```python
from build123d import *

# Parameters (mm, degrees)
F0_W     = 40
F0_H     = 20
F1_DEPTH = 10
F2_W     = 9.5
F2_H     = 8.5
F3_DEPTH = 10
F4_R     = 2
F5_DEPTH = 10
F6_W     = 40
F6_H     = 2
F7_DEPTH = 3


with BuildPart() as f1:
    # F0 (on Top) → F1 (new body)
    with BuildSketch(Plane.XY):
        Rectangle(F0_W, F0_H)
    extrude(amount=F1_DEPTH)

    # F2 (on face) → F3 (join)
    with BuildSketch(Plane.XY.offset(10)):
        with Locations((0, -5.75)):
            Rectangle(F2_W, F2_H)
    extrude(amount=F3_DEPTH)

    # F4 (on face) → F5 (cut)
    with BuildSketch(Plane.XZ.offset(10)):
        with Locations((0, 15)):
            Circle(F4_R)
    extrude(amount=-F5_DEPTH, mode=Mode.SUBTRACT)

    # F6 (on face) → F7 (cut)
    with BuildSketch(Plane(origin=(0, 10, 0), x_dir=(-1, 0, 0), z_dir=(0, 1, 0))):
        with Locations((0, 4.25)):
            Rectangle(F6_W, F6_H)
    extrude(amount=-F7_DEPTH, mode=Mode.SUBTRACT)


solid = f1.part
```
Work out the finished part from the listing and answer in its coordinate system (mm). A direction names the side the tool comes from. Round coordinates to 2 decimals unless told otherwise and drop trailing zeros. Write each loop counter-clockwise with the first axis right and the second up, starting at its lowest first coordinate (ties: lowest second). Pieces come first, ordered by that corner, then holes. Notation, with made-up numbers: (20, 42) -> (78, 42) arc R5 ccw to (78, 51) -> close; hole circle Ø9 at (-20, 51.5). An arc over 180 degrees is marked (long way). Write each question's results on one line, items separated by ' | '.
1) For a pull along Z with two mould halves and no side action, classify faces 1 (the flat face through (-4.75, -6, 15)), 2 (the flat face through (0, -6, 20)), 3 (the flat face through (0, 9, 5.25)), 4 (the flat face through (0, 0, 0)) as +Z half, -Z half, draft (parallel to the pull), parting line (faces both ways), or undercut.
Findings:
face 1: draft | face 2: +Z half | face 3: undercut | face 4: -Z half
2) Which of the six approach directions +Z, -Z, +X, -X, +Y, -Y give full straight-line access (tool end or side, diameter ignored) to faces 5 (the flat face through (0, 9, 3.25)), 6 (the flat face through (-2.2, -1.5, 14.9)), 7 (the flat face through (4.75, -6, 15))?
Findings:
face 5: +X, -X, +Y | face 6: +Z, +X, -X, +Y | face 7: +Z, +X, +Y, -Y
3) The part is cut by section A-A (x = 0). Write down the section's boundary in (y, z), and give its area (3 significant figures).
Findings:
outline: (-10, 0) -> (10, 0) -> (10, 3.25) -> (7, 3.25) -> (7, 5.25) -> (10, 5.25) -> (10, 10) -> (-1.5, 10) -> (-1.5, 13) -> (-10, 13) -> close; (-10, 17) -> (-1.5, 17) -> (-1.5, 20) -> (-10, 20) -> close | area: 245 mm²
4) Flat-ended cylindrical pins translate along their axes: pin 1 (7.5 mm diameter, centred on x = 0, z = 15, fed in from +Y); pin 2 (2.5 mm diameter, centred on x = 4, y = 8, fed in from +Z); pin 3 (7 mm diameter, centred on y = -7, z = 14.5, fed in from +X). Find the tip coordinate at first contact, or state that the pin passes through.
Findings:
pin 1: stops at y = -1.5 | pin 2: stops at z = 10 | pin 3: stops at x = 4.75
5) The part is cut by section D-D (x = 16). Write down the section's boundary in (y, z).
Findings:
outline: (-10, 0) -> (10, 0) -> (10, 3.25) -> (7, 3.25) -> (7, 5.25) -> (10, 5.25) -> (10, 10) -> (-10, 10) -> close
6) The part is cut by section B-B (y = -6.25). Write down the section's boundary in (x, z).
Findings:
outline: (-20, 0) -> (20, 0) -> (20, 10) -> (4.75, 10) -> (4.75, 20) -> (-4.75, 20) -> (-4.75, 10) -> (-20, 10) -> close; hole circle Ø4 at (0, 15)
7) Consider line 1 along Z through (x, y) = (0, -4); line 2 along Z through (x, y) = (-17, 8.25); line 3 along Y through (x, z) = (-9, 4.25). Determine where each line is inside the solid, lowest interval first. Write a range as [from, to].
Findings:
line 1: z = [0, 13], [17, 20] | line 2: z = [0, 3.25], [5.25, 10] | line 3: y = [-10, 7]
8) The part is cut by section C-C (z = 15). Write down the section's boundary in (x, y), and give its area (4 significant figures).
Findings:
outline: (-4.75, -10) -> (-2, -10) -> (-2, -1.5) -> (-4.75, -1.5) -> close; (2, -10) -> (4.75, -10) -> (4.75, -1.5) -> (2, -1.5) -> close | area: 46.75 mm²
